Source: CAD feature listing. Evaluate the final solid. Frame: model axes, mm. Face numbers are marked on the shaded views. A direction names the side the tool comes from. Give positions to 0.01 mm unless a question says otherwise; leave off trailing zeros. Write each loop counter-clockwise with the first axis right and the second up, starting at its lowest first coordinate (ties: lowest second). Pieces come first, ordered by that corner, then holes. Notation, with made-up numbers: (19, -22.5) -> (38, -22.5) arc R9 cw to (38, -9.5) -> close; hole circle Ø1 at (73, -33). An arc over 180 degrees is marked (long way). Use a Markdown table: item, result. Add a question column.
```python
from build123d import *

# Parameters (mm, degrees)
SZKIC1_R                    = 2.85
SZKIC1_R_2                  = 1.6
DODANIE_WYCI_GNI_CIE1_DEPTH = 1
DODANIE_WYCI_GNI_CIE2_DEPTH = 0.7
SZKIC3_W                    = 5.7
SZKIC3_H                    = 1
DODANIE_WYCI_GNI_CIE3_DEPTH = 2


with BuildPart() as part:
    # Szkic1 → Dodanie-wyciągnięcie1 (new body)
    with BuildSketch(Plane.XY):
        Circle(SZKIC1_R)
        Circle(SZKIC1_R_2, mode=Mode.SUBTRACT)
    extrude(amount=DODANIE_WYCI_GNI_CIE1_DEPTH)

    # Szkic2 → Dodanie-wyciągnięcie2 (add)
    with BuildSketch(Plane.XY.offset(1)):
        with BuildLine():
            Line((2.85, 5.75), (0, 5.75))
            Line((0, 5.75), (-2.85, 5.75))
            Line((-2.85, 5.75), (-2.85, 0))
            ThreePointArc((-2.85, 0), (0, -2.85), (2.85, 0))
            Line((2.85, 0), (2.85, 5.75))
        make_face()
        with BuildLine():
            ThreePointArc((1.6, 0), (-1.13137085, -1.13137085), (0, 1.6))
            ThreePointArc((0, 1.6), (1.13137085, 1.13137085), (1.6, 0))
        make_face(mode=Mode.SUBTRACT)
    extrude(amount=DODANIE_WYCI_GNI_CIE2_DEPTH)

    # Szkic3 → Dodanie-wyciągnięcie3 (add)
    with BuildSketch(Plane(origin=(0, 0, 1), x_dir=(-1, 0, 0), z_dir=(0, 0, -1))):
        with Locations((0, 5.25)):
            Rectangle(SZKIC3_W, SZKIC3_H)
    extrude(amount=DODANIE_WYCI_GNI_CIE3_DEPTH)


solid = part.part
```
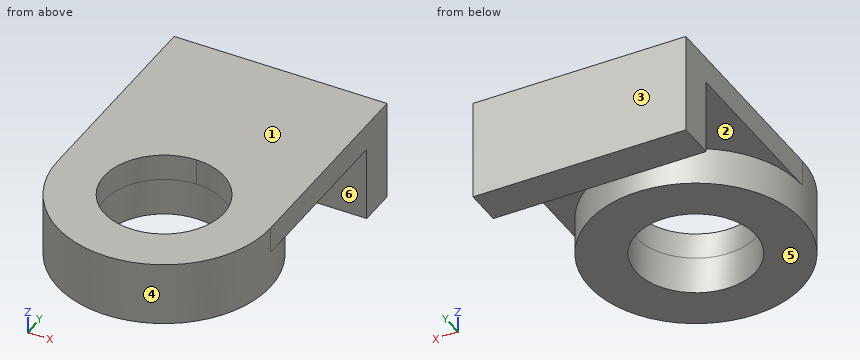
(1) Cut plane C-C on z = 1.2. Return the cut outline in (x, y), then the cut area to 3 significant figures.
(2) Material intervals for L1, parallel to Y at x = 0, z = 0.8; L2, parallel to X at y = 0, z = 1.55; L3, parallel to Y at x = 1.35, z = 0.9, sorted ascending.
(3) First-contact query: pin 1 Ø1.9 at (x, y) = (0, 0) entering from -Z; pin 2 Ø2 at (x, y) = (-1, 0) entering from -Z. Flat tips, straight axial feed; report the tip coordinate or a pass-through.
(4) Access query for the marked faces 4, 5 and 6. Directions: +Z, -Z, +X, -X, +Y, -Y. A direction counts if a zero-diameter tool reaches every point of the face in a straight line with its end or side. Return the directions, or none.
(5) Cut plane A-A on z = 0.5. Return the cut outline in (x, y).
(6) Cut plane B-B on x = 1.2. Return the cut outline in (y, z).
(7) Mould query, pull axis Y, two halves, no side actions, for the marked faces 1, 2 and 3. Classes: +Y half, -Y half, draft (parallel to the pull), parting line (faces both ways), or undercut.
(8) Cut plane D-D on y = 0.5. Return the cut outline in (x, z), then the cut area to 3 significant figures.
Output:
| question | item | result |
|---|---|---|
| 1 | outline | (-2.85, 0) arc R2.85 ccw to (2.85, 0) -> (2.85, 5.75) -> (-2.85, 5.75) -> close; hole circle Ø3.2 at (0, 0) |
| 1 | area | 37.5 mm^2 |
| 2 | L1 | -2.85 to -1.6, 1.6 to 2.85, 4.75 to 5.75 |
| 2 | L2 | -2.85 to -1.6, 1.6 to 2.85 |
| 2 | L3 | -2.51 to -0.86, 0.86 to 2.51, 4.75 to 5.75 |
| 3 | pin 1 | through |
| 3 | pin 2 | z = 0 |
| 4 | face 4 | -Z |
| 4 | face 5 | -Z, +X, -X, -Y |
| 4 | face 6 | -Z, +X, -X |
| 5 | outline | circle Ø5.7 at (0, 0); (-2.85, 4.75) -> (2.85, 4.75) -> (2.85, 5.75) -> (-2.85, 5.75) -> close; hole circle Ø3.2 at (0, 0) |
| 6 | outline | (-2.59, 0) -> (-1.06, 0) -> (-1.06, 1.7) -> (-2.59, 1.7) -> close; (1.06, 0) -> (2.59, 0) -> (2.59, 1) -> (4.75, 1) -> (4.75, -1) -> (5.75, -1) -> (5.75, 1.7) -> (1.06, 1.7) -> close |
| 7 | face 1 | draft |
| 7 | face 2 | undercut |
| 7 | face 3 | +Y half |
| 8 | outline | (-2.85, 1) -> (-2.81, 1) -> (-2.81, 0) -> (-1.52, 0) -> (-1.52, 1.7) -> (-2.85, 1.7) -> close; (1.52, 0) -> (2.81, 0) -> (2.81, 1) -> (2.85, 1) -> (2.85, 1.7) -> (1.52, 1.7) -> close |
| 8 | area | 4.43 mm^2 |
